```python
from build123d import *
from build123d import SkipClean  # not in build123d's __all__

# Parameters (mm, degrees)
F1_DEPTH = 20
F3_DEPTH = 50
F5_DEPTH = 5
F7_DEPTH = 25


# Not quite as in the source:
# - after a boolean that leaves OpenCascade's solid faulty, fix() repairs it


with BuildPart() as f1:
    # F0 (on Front) → F1 (new body)
    with BuildSketch(Plane.XZ):
        with BuildLine():
            ThreePointArc((0, -10), (7.0710678119, -7.0710678119), (10, 0))
            ThreePointArc((10, 0), (7.0710678119, 7.0710678119), (0, 10))
            ThreePointArc((0, 10), (-10, 0), (0, -10))
        make_face()
        with BuildLine():
            ThreePointArc((0, 10), (7.0710678119, 7.0710678119), (10, 0))
            ThreePointArc((10, 0), (7.0710678119, -7.0710678119), (0, -10))
            Line((0, -10), (15, -10))
            Line((15, -10), (20, -5))
            Line((20, -5), (20, 5))
            Line((20, 5), (15, 10))
            Line((15, 10), (0, 10))
        make_face()
    extrude(amount=F1_DEPTH)

    # F2 (on face) → F3 (cut)
    with BuildSketch(Plane.YZ.offset(20)):
        Polygon((-20, 2.5), (-20, 0), (-20, -2.5), (-10, -2.5), (-10, 2.5), align=None)
    extrude(amount=-F3_DEPTH, mode=Mode.SUBTRACT)

    # F4 (on face) → F5 (cut)
    with BuildSketch(Plane.XZ.offset(20)):
        with BuildLine():
            ThreePointArc((9.6824583655, -2.5), (6.123724357, -7.9056941504), (0, -10))
            Line((0, -10), (15, -10))
            Line((15, -10), (20, -5))
            Line((20, -5), (20, -2.5))
            Line((20, -2.5), (9.6824583655, -2.5))
        make_face()
        with BuildLine():
            Line((15, 10), (0, 10))
            ThreePointArc((0, 10), (6.123724357, 7.9056941504), (9.6824583655, 2.5))
            Line((9.6824583655, 2.5), (20, 2.5))
            Line((20, 2.5), (20, 5))
            Line((20, 5), (15, 10))
        make_face()
    with SkipClean():  # cleaning this boolean's faces spoils the solid; the shape is the same uncleaned
        extrude(amount=-F5_DEPTH, mode=Mode.SUBTRACT)

    # F6 (on face) → F7 (cut)
    with BuildSketch(Plane.XZ.offset(20)):
        with BuildLine():
            ThreePointArc((-4.3301270189, 2.5), (-1.2940952255, -4.8296291314), (5, 0))
            ThreePointArc((5, 0), (4.8296291314, 1.2940952255), (4.3301270189, 2.5))
            Line((4.3301270189, 2.5), (-4.3301270189, 2.5))
        make_face()
        with BuildLine():
            Line((-4.3301270189, 2.5), (4.3301270189, 2.5))
            ThreePointArc((4.3301270189, 2.5), (0, 5), (-4.3301270189, 2.5))
        make_face()
    extrude(amount=-F7_DEPTH, mode=Mode.SUBTRACT)

    add(f1.part.fix(), mode=Mode.REPLACE)


solid = f1.part
```
CAD build for the part. Positions are in the model's coordinates, mm. A direction names the side the tool comes from. Coordinates: 2 decimals unless noted, no trailing zeros. Order: outer loops, then holes, each group sorted by start corner. A loop starts at its lowest first (then second) coordinate and runs counter-clockwise, first axis right, second up. Notation, with made-up numbers: M 34,83.5 L 92,83.5 A22 ccw 92,118.5 Z; hole C -37.75,0.25 d4. An arc over 180 degrees is marked long. Write each question's results on one line, items separated by ' | '. Start each with the question number.
Q1. Cut at A-A (y = -17.25). List the corners of the cut face in (x, z).
Q2. Cut at D-D (y = -7.75). List the corners of the cut face in (x, z), then the cut area to 3 significant figures.
Q3. Which spindle directions (+Z, -Z, +X, -X, +Y, -Y) get a long thin tool onto all of the face, cutting with end or side? Do faces 1 (the flat face through (12, -15, -6)), 2 (the flat face through (12, -10, 0)), 3 (the flat face through (12, -15, 6)). Say none if no direction does.
Q4. Pull direction Z, two halves, no side cores. Call faces 4 (the flat face through (8, -7, 10)), 5 (the flat face through (0, -20, -6)), 6 (the flat face through (-7, -15, 2.5)), 7 (the flat face through (7, -7, -10)): +Z half, -Z half, draft (parallel to the pull), parting line (faces both ways), or undercut.
Q5. Cut at C-C (z = 1). List the corners of the cut face in (x, y).
Q6. Drill centre lines: probe 1 along X at (y, z) = (-6, 0); probe 2 along Z at (x, y) = (0, -5.75); probe 3 along Z at (x, y) = (-3.5, -10.5). Where is each one in solid material? Low to high. Write a range as from..to.
Q7. Cut at B-B (x = 10.5). List the corners of the cut face in (y, z).
Q8. Flat gauge pins, fed straight in: P1, Ø5, axis at x = -5, y = -11.5, coming from the -Z side; P2, Ø6, axis at x = -7.5, y = -13, coming from the +Z side; P3, Ø1, axis at x = 3.5, y = -16, coming from the -Z side; P4, Ø6, axis at x = 0, z = 0, coming from the +Y side. Where does each tip first touch, or does it go through?
Found:
1) outline: M -9.68,-2.5 A10 ccw 9.68,-2.5 L 4.33,-2.5 A5 cw -4.33,-2.5 Z; M -9.68,2.5 L -4.33,2.5 A5 cw 4.33,2.5 L 9.68,2.5 A10 ccw Z
2) outline: M 0,-10 L 15,-10 L 20,-5 L 20,5 L 15,10 L 0,10 A10 ccw Z; hole C 0,0 d10 | area: 454 mm²
3) face 1: -Z, +X, -Y | face 2: +X, -X, -Y | face 3: +Z, +X, -Y
4) face 4: +Z half | face 5: draft | face 6: undercut | face 7: -Z half
5) outline: M -9.95,-10 L -4.9,-10 L -4.9,0 L -9.95,0 Z; M 4.9,-10 L 20,-10 L 20,0 L 4.9,0 Z
6) probe 1: -10..-5, 5..20 | probe 2: -10..-5, 5..10 | probe 3: -9.37..-3.57, 3.57..9.37
7) outline: M -15,-10 L 0,-10 L 0,10 L -15,10 L -15,2.5 L -10,2.5 L -10,-2.5 L -15,-2.5 Z
8) P1: z = -9.68 | P2: z = 8.93 | P3: z = -9.54 | P4: through
